Can you work these out from the model? Positions are in its coordinate system, mm. A direction names the side the tool comes from. Round coordinates to 2 decimals unless told otherwise and drop trailing zeros. Loops run counter-clockwise (first coordinate to the right, second up) from the corner with the lowest first, then second, coordinate; pieces in that order, holes last. Notation, with made-up numbers: (87, -26.5) -> (98, -26.5) arc R24 cw to (98, -6.5) -> close; hole circle Ø7 at (16.25, -35). An arc over 180 degrees is marked (long way). Answer as a JSON object with one key per item and string values.
```python
from build123d import *

# Parameters (mm, degrees)
SALIENTE_EXTRUIR1_DEPTH = 10.1
CROQUIS4_W              = 20
CROQUIS4_H              = 1.2
CORTAR_EXTRUIR1_DEPTH   = 10
SALIENTE_EXTRUIR2_START = -7.7
SALIENTE_EXTRUIR2_DEPTH = 7.7
CROQUIS6_R              = 2.5
CORTAR_EXTRUIR2_DEPTH   = 1.5
CROQUIS7_R              = 2.05
CORTAR_EXTRUIR3_DEPTH   = 0.5


with BuildPart() as part:
    # Croquis3 → Saliente-Extruir1 (new body)
    with BuildSketch(Plane(origin=(0, 0, 0), x_dir=(1, 0, 0), z_dir=(0, 1, 0))):
        with BuildLine():
            Line((33.362812396, -5.019964628), (-32.868233457, -5.019964628))
            Line((-32.868233457, -5.019964628), (-32.868233457, 4.980035372))
            Line((-32.868233457, 4.980035372), (33.131766543, 4.980035372))
            ThreePointArc((33.131766543, 4.980035372), (46.332773431, 0.282370053), (33.362812396, -5.019964628))
        make_face()
    extrude(amount=SALIENTE_EXTRUIR1_DEPTH)

    # Croquis4 → Cortar-Extruir1 (cut)
    with BuildSketch(Plane.XY.offset(5.019964628)):
        with Locations((-22.868233457, 9.5)):
            Rectangle(CROQUIS4_W, CROQUIS4_H)
    cortar_extruir1 = extrude(amount=-CORTAR_EXTRUIR1_DEPTH, mode=Mode.SUBTRACT)

    # Simetría1: Cortar-Extruir1 across plane
    add(cortar_extruir1.mirror(Plane.ZX.offset(5.05)), mode=Mode.SUBTRACT)

    # Croquis5 → Saliente-Extruir2 (add)
    with BuildSketch(Plane(origin=(0, 8.9, 0), x_dir=(1, 0, 0), z_dir=(0, 1, 0)).offset(SALIENTE_EXTRUIR2_START)):
        with BuildLine():
            Line((-32.868233457, 4.980035372), (-32.868233457, -5.019964628))
            ThreePointArc((-32.868233457, -5.019964628), (-39.493870843, -3.678231071), (-44.60405989, 0.747295745))
            ThreePointArc((-44.60405989, 0.747295745), (-42.906522418, 7.611577683), (-36.04224048, 5.914040211))
            ThreePointArc((-36.04224048, 5.914040211), (-34.577950006, 5.030024916), (-32.868233457, 4.980035372))
        make_face()
    extrude(amount=SALIENTE_EXTRUIR2_DEPTH)

    # Croquis6 → Cortar-Extruir2 (cut)
    with BuildSketch(Plane(origin=(0, 8.9, 0), x_dir=(1, 0, 0), z_dir=(0, 1, 0))):
        with Locations(Location((-40.323150185, 3.330667978, 0), (0, 0, 270))):
            Circle(CROQUIS6_R)
    cortar_extruir2 = extrude(amount=-CORTAR_EXTRUIR2_DEPTH, mode=Mode.SUBTRACT)

    # Simetría2: Cortar-Extruir2 across plane
    add(cortar_extruir2.mirror(Plane.ZX.offset(5.05)), mode=Mode.SUBTRACT)

    # Croquis7 → Cortar-Extruir3 (cut)
    with BuildSketch(Plane(origin=(0, 10.1, 0), x_dir=(1, 0, 0), z_dir=(0, 1, 0))):
        with Locations(Location((38.834774462, 0.109131896, 0), (0, 0, 270))):
            Circle(CROQUIS7_R)
    extrude(amount=-CORTAR_EXTRUIR3_DEPTH, mode=Mode.SUBTRACT)


solid = part.part
```
Q1. I want a section at D-D, the plane z = -3.75. Write out the boundary of the cut face in (x, y).
Determined:
{"outline": "(-45.31, 1.2) -> (-42.79, 1.2) -> (-42.79, 2.7) -> (-37.86, 2.7) -> (-37.86, 1.2) -> (-12.87, 1.2) -> (-12.87, 0) -> (45.39, 0) -> (45.39, 10.1) -> (-12.87, 10.1) -> (-12.87, 8.9) -> (-37.86, 8.9) -> (-37.86, 7.4) -> (-42.79, 7.4) -> (-42.79, 8.9) -> (-45.31, 8.9) -> close"}
Q2. If I drill on L1, parallel to Z at x = -29, y = 4.75; L2, parallel to X at y = 8.25, z = -4.5; L3, parallel to Y at x = -31, z = 0.25, over which ranges is the centre line in solid material (lowest first)? Write a range as [from, to].
Determined:
{"L1": "[-4.98, 5.02]", "L2": "[-45.18, -42.53], [-38.11, 44.92]", "L3": "[1.2, 8.9]"}
Q3. I want a section at A-A, the plane x = -31. Write out the boundary of the cut face in (y, z), then the cut area to 3 significant figures.
Determined:
{"outline": "(1.2, -4.98) -> (8.9, -4.98) -> (8.9, 5.02) -> (1.2, 5.02) -> close", "area": "77.0 mm²"}
Q4. I want a section at C-C, the plane x = 28. Write out the boundary of the cut face in (y, z).
Determined:
{"outline": "(0, -4.98) -> (10.1, -4.98) -> (10.1, 5.02) -> (0, 5.02) -> close"}
Q5. On a 3-axis mill with a long thin cutter (end or side, diameter ignored), from which of +Z, -Z, +X, -X, +Y, -Y can I reach the whole of each face in a straight line? I mean faces 1 (the flat face through (-40, 7.4, -3)), 2 (the flat face through (-29, 1.2, 0)), 3 (the flat face through (-40, 2.7, -3)). Say none if no direction works.
Determined:
{"face 1": "+Y", "face 2": "+Z, -Z, -X, -Y", "face 3": "-Y"}
Q6. I want a section at B-B, the plane z = 0.75. Write out the boundary of the cut face in (x, y).
Determined:
{"outline": "(-43.41, 1.2) -> (-12.87, 1.2) -> (-12.87, 0) -> (46.29, 0) -> (46.29, 10.1) -> (40.7, 10.1) -> (40.7, 9.6) -> (36.97, 9.6) -> (36.97, 10.1) -> (-12.87, 10.1) -> (-12.87, 8.9) -> (-43.41, 8.9) -> close"}
Q7. I'm going to push flat-ended pins straight in: pin 1 (8 mm diameter, centred on x = -40.32, z = -3.33, fed in from +Y); pin 2 (4 mm diameter, centred on x = -22.5, z = -2.5, fed in from -Y); pin 3 (1.3 mm diameter, centred on y = 1, z = 0, fed in from -X). Where does each tip first touch, or does it pass through?
Determined:
{"pin 1": "y = 8.9", "pin 2": "y = 1.2", "pin 3": "x = -44.51"}
Q8. We'd pull the mould along X, two halves only. Please class faces 4 (the cylindrical face through (-42.764, 1.939, -3.873)), 5 (the flat face through (-29, 8.9, 0)): pulls with the +X half, pulls with the -X half, needs draft (parallel to the pull), parting line crosses it, or undercut.
Determined:
{"face 4": "undercut", "face 5": "needs draft"}
